Verification items for the finished model (mm, model axes). A direction names the side the tool comes from. Coordinates: 2 decimals unless noted, no trailing zeros. Write each loop counter-clockwise with the first axis right and the second up, starting at its lowest first coordinate (ties: lowest second). Pieces come first, ordered by that corner, then holes.
```python
from build123d import *

# Parameters (mm, degrees)
SKETCH3_W           = 200
SKETCH3_H           = 130
BOSS_EXTRUDE1_DEPTH = 300
SHELL2_T            = -5
SKETCH12_R          = 5
CUT_EXTRUDE1_DEPTH  = 300
SKETCH13_R          = 5
CUT_EXTRUDE3_DEPTH  = 300


with BuildPart() as part:
    # Sketch3 → Boss-Extrude1 (new body)
    with BuildSketch(Plane(origin=(0, 0, 0), x_dir=(0, 0, -1), z_dir=(1, 0, 0))):
        with Locations((-81.156140409, 58.885017422)):
            Rectangle(SKETCH3_W, SKETCH3_H)
    extrude(amount=BOSS_EXTRUDE1_DEPTH)

    # Shell2
    shell2_openings = [part.faces().sort_by_distance(p)[0] for p in [
        (0, 58.885017422, 81.156140409),
        (150, -6.114982578, 81.156140409),
    ]]
    offset(amount=SHELL2_T, openings=shell2_openings, kind=Kind.INTERSECTION)

    # Sketch12 → Cut-Extrude1 (cut)
    with BuildSketch(Plane(origin=(0, 0, -18.843859591), x_dir=(-1, 0, 0), z_dir=(0, 0, -1))):
        with Locations((-288.794979597, 65)):
            Circle(SKETCH12_R)
    extrude(amount=-CUT_EXTRUDE1_DEPTH, mode=Mode.SUBTRACT)

    # Sketch13 → Cut-Extrude3 (cut)
    with BuildSketch(Plane.XY.offset(181.156140409)):
        with Locations(Location((7.10538066, 65, 0), (0, 0, 270))):
            Circle(SKETCH13_R)
    extrude(amount=-CUT_EXTRUDE3_DEPTH, mode=Mode.SUBTRACT)


solid = part.part
```
1. Sectioned sample at D-D, the plane z = 64. Record the boundary of the cut face in (x, y).
2. Tool access check on faces 1 (the flat face through (148, 58, 181.156)), 2 (the flat face through (145, 56, -13.844)). Record the directions out of +Z, -Z, +X, -X, +Y, -Y that give a thin tool (end or side, any length) a straight path to the whole face; none if there is none.
3. Sectioned sample at A-A, the plane y = 65. Record the boundary of the cut face in (x, z).
4. Gauge pin test, flat ends, axial feed: P1, Ø8, axis at y = 76.5, z = 11.5, coming from the -X side; P2, Ø8, axis at x = 7.11, y = 65, coming from the -Z side. Record the tip position at first contact, or that the pin passes through.
5. Material ranges on L1, parallel to Z at x = 161, y = 42; L2, parallel to X at y = 44, z = 86; L3, parallel to Y at x = 60, z = 32, recorded low to high.
6. Sectioned sample at C-C, the plane y = 103.5. Record the boundary of the cut face in (x, z), and give its area (3 significant figures).
7. Draft check along Z on faces 3 (the flat face through (295, 57, 82)), 4 (the flat face through (148, 58, -18.844)), 5 (the flat face through (0, 122, 82)). Enter one of: pulls with the +Z half, pulls with the -Z half, needs draft (parallel to the pull), parting line crosses it, or undercut.
8. Sectioned sample at B-B, the plane x = 234. Record the boundary of the cut face in (y, z), and give its area (3 significant figures).
Outcome:
1. outline: (0, 118.89) - (295, 118.89) - (295, -6.11) - (300, -6.11) - (300, 123.89) - (0, 123.89) - close
2. face 1: +Z, +X, -X, +Y, -Y
2. face 2: -X, -Y
3. outline: (0, -18.84) - (2.11, -18.84) - (2.11, -13.84) - (0, -13.84) - close; (0, 176.16) - (2.11, 176.16) - (2.11, 181.16) - (0, 181.16) - close; (12.11, -18.84) - (283.79, -18.84) - (283.79, -13.84) - (12.11, -13.84) - close; (12.11, 176.16) - (283.79, 176.16) - (283.79, 181.16) - (12.11, 181.16) - close; (293.79, -18.84) - (300, -18.84) - (300, 181.16) - (293.79, 181.16) - (293.79, 176.16) - (295, 176.16) - (295, -13.84) - (293.79, -13.84) - close
4. P1: stops at x = 295
4. P2: passes through
5. L1: z = -18.84 to -13.84, 176.16 to 181.16
5. L2: x = 295 to 300
5. L3: y = 118.89 to 123.89
6. outline: (0, -18.84) - (300, -18.84) - (300, 181.16) - (0, 181.16) - (0, 176.16) - (295, 176.16) - (295, -13.84) - (0, -13.84) - close
6. area: 3,950 mm2
7. face 3: undercut
7. face 4: pulls with the -Z half
7. face 5: needs draft
8. outline: (-6.11, -18.84) - (123.89, -18.84) - (123.89, 181.16) - (-6.11, 181.16) - (-6.11, 176.16) - (118.89, 176.16) - (118.89, -13.84) - (-6.11, -13.84) - close
8. area: 2,250 mm2
